The model under review builds one solid part; all positions refer to its coordinate system, in mm. A direction names the side the tool comes from. Round coordinates to 2 decimals unless told otherwise and drop trailing zeros. Write each loop counter-clockwise with the first axis right and the second up, starting at its lowest first coordinate (ties: lowest second). Pieces come first, ordered by that corner, then holes. Notation, with made-up numbers: (16, -31.5) - (75, -31.5) arc R27 ccw to (75, -7.5) - close; hole circle Ø2 at (-20, 51.25). An arc over 180 degrees is marked (long way). Use one line per item in the form item = value.
from build123d import *

# Parameters (mm, degrees)
BOSS_EXTRUDE1_DEPTH      = 2.54
SKETCH2_W                = 9.525
SKETCH2_H                = 38.1
BOSS_EXTRUDE2_DEPTH      = 15.875
BOSS_EXTRUDE3_DEPTH      = 5.08
M3_CLEARANCE_HOLE1_D     = 3.3
M3_CLEARANCE_HOLE1_DEPTH = 12.7
M3_CLEARANCE_HOLE1_TIP   = 0.991420021
SKETCH7_W                = 35.71875
SKETCH7_H                = 2.38125
CUT_EXTRUDE1_DEPTH       = 2.54
FILLET1_R                = 1.27
SKETCH8_R                = 3.4925
CUT_EXTRUDE2_DEPTH       = 10.16
CUT_EXTRUDE3_DEPTH       = 57.171484091
CUT_EXTRUDE3_DEPTH_BACK  = 57.171484091
SKETCH9_W                = 10.431111816
SKETCH9_H                = 47.706198334
FILLET3_R                = 1.27


with BuildPart() as part:
    # Sketch1 → Boss-Extrude1 (new body)
    with BuildSketch(Plane(origin=(0, 0, 0), x_dir=(1, 0, 0), z_dir=(0, 1, 0))):
        Polygon((0, 0), (38.1, 0), (38.1, 2.38125), (2.38125, 2.38125), (2.38125, 38.1), (0, 38.1), align=None)
    extrude(amount=BOSS_EXTRUDE1_DEPTH)

    # Sketch2 → Boss-Extrude2 (add)
    with BuildSketch(Plane(origin=(0, 2.54, 0), x_dir=(1, 0, 0), z_dir=(0, 1, 0))):
        with Locations((-4.7625, 19.05)):
            Rectangle(SKETCH2_W, SKETCH2_H)
        Polygon((0, 0), (-9.525, 0), (-9.525, -9.525), (38.1, -9.525), (38.1, 0), align=None)
    extrude(amount=-BOSS_EXTRUDE2_DEPTH)

    # Sketch3 → Boss-Extrude3 (add)
    with BuildSketch(Plane(origin=(0, -13.335, 0), x_dir=(-1, 0, 0), z_dir=(0, -1, 0))):
        Polygon((9.525, -9.525), (-38.1, -9.525), (-38.1, 18.373079092), (-18.373079092, 38.1), (9.525, 38.1), align=None)
    extrude(amount=BOSS_EXTRUDE3_DEPTH)

    # M3 Clearance Hole1
    with Locations(Plane(origin=(0, -18.415, 0), x_dir=(-1, 0, 0), z_dir=(0, -1, 0))):
        with Locations((-10, 32.5), (-32.5, 10)):
            Hole(M3_CLEARANCE_HOLE1_D / 2, depth=M3_CLEARANCE_HOLE1_DEPTH)
            with Locations((0, 0, -(M3_CLEARANCE_HOLE1_DEPTH + M3_CLEARANCE_HOLE1_TIP / 2))):  # 118° drill point
                Cone(0, M3_CLEARANCE_HOLE1_D / 2, M3_CLEARANCE_HOLE1_TIP, mode=Mode.SUBTRACT)

    # Sketch7 → Cut-Extrude1 (cut)
    with BuildSketch(Plane(origin=(0, 2.54, 0), x_dir=(1, 0, 0), z_dir=(0, 1, 0))):
        with Locations((20.240625, 1.190625)):
            Rectangle(SKETCH7_W, SKETCH7_H)
        Polygon((0, 0), (2.38125, 0), (2.38125, 2.38125), (2.38125, 38.1), (0, 38.1), align=None)
    extrude(amount=-CUT_EXTRUDE1_DEPTH, mode=Mode.SUBTRACT)

    # Fillet1
    fillet1_edges = [part.edges().sort_by_distance(p)[0] for p in [
        (38.1, 2.54, 4.7625),
        (0, -5.3975, -38.1),
        (-9.525, -7.9375, -38.1),
        (38.1, -5.3975, 0),
        (14.2875, 2.54, 9.525),
        (38.1, -7.9375, 9.525),
        (-9.525, -7.9375, 9.525),
        (-9.525, 2.54, -14.2875),
        (-9.525, -18.415, -14.2875),
        (14.2875, -18.415, 9.525),
        (-4.7625, 2.54, -38.1),
        (0, 2.54, -19.05),
        (19.05, 2.54, 0),
    ]]
    fillet(fillet1_edges, radius=FILLET1_R)

    # Sketch8 → Cut-Extrude2 (cut)
    with BuildSketch(Plane(origin=(0, -13.335, 0), x_dir=(1, 0, 0), z_dir=(0, 1, 0))):
        with Locations(Location((10, 32.5, 0), (0, 0, 270))):
            Circle(SKETCH8_R)
    extrude(amount=-CUT_EXTRUDE2_DEPTH, mode=Mode.SUBTRACT)

    # Sketch9 → Cut-Extrude3 (cut, two sides: drawn at the far end of the back side and taken through both)
    with BuildSketch(Plane(origin=(0, -13.335, 0), x_dir=(1, 0, 0), z_dir=(0, 1, 0)).offset(-CUT_EXTRUDE3_DEPTH_BACK)):
        with Locations((-9.978055908, 11.071900833)):
            Rectangle(SKETCH9_W, SKETCH9_H)
        Polygon((25.888370715, 34.925), (25.888370715, 38.1), (18.373079092, 38.1), (21.548079092, 34.925), align=None)
        with BuildLine():
            Line((21.548079092, 34.925), (18.373079092, 38.1))
            Line((18.373079092, 38.1), (-1.27, 38.1))
            ThreePointArc((-1.27, 38.1), (-0.371974388, 37.728025612), (0, 36.83))
            Line((0, 36.83), (0, 34.925))
            Line((0, 34.925), (7.486649398, 34.925))
            ThreePointArc((7.486649398, 34.925), (10, 35.9925), (12.513350602, 34.925))
            Line((12.513350602, 34.925), (21.548079092, 34.925))
        make_face()
        with BuildLine():
            ThreePointArc((0, 36.83), (-0.371974388, 37.728025612), (-1.27, 38.1))
            Line((-1.27, 38.1), (-15.193611816, 38.1))
            Line((-15.193611816, 38.1), (-15.193611816, 34.925))
            Line((-15.193611816, 34.925), (-4.7625, 34.925))
            Line((-4.7625, 34.925), (0, 34.925))
            Line((0, 34.925), (0, 36.83))
        make_face()
    extrude(amount=CUT_EXTRUDE3_DEPTH + CUT_EXTRUDE3_DEPTH_BACK, mode=Mode.SUBTRACT)

    # Fillet3
    fillet3_edges = [part.edges().sort_by_distance(p)[0] for p in [
        (-4.7625, 2.168025612, 9.153025612),
        (-4.7625, -7.9375, 9.525),
        (-0.371974388, 2.168025612, -34.925),
        (-3.01625, 2.54, -34.925),
        (-4.7625, -18.415, -13.335),
        (0, -6.0325, -34.925),
        (-4.7625, -18.043025612, 9.153025612),
        (-4.7625, -7.9375, -34.925),
        (-4.7625, 2.54, -13.335),
    ]]
    fillet(fillet3_edges, radius=FILLET3_R)


solid = part.part
(1) Insertion check: P1, Ø4.5, axis at x = 32.5, z = -10, coming from the +Y side (3 decimals); P2, Ø10, axis at y = -9.5, z = -28, coming from the +X side; P3, Ø2, axis at y = -13, z = -6.5, coming from the +X side; P4, Ø6.5, axis at x = 10, z = -32.5, coming from the -Y side. Each pin has a flat end and moves straight along its axis. Give the tip position at first contact, or say it passes through.
Geometry results:
P1 = -13.335
P2 = 31.68
P3 = 38.1
P4 = through
(2) Add section D-D on y = -4.5. Write out the cut boundary in (x, z) (1 decimal), then the cut area to 3 significant figures.
Geometry results:
outline = (-4.8, -33.7) arc R1.3 ccw to (-3.5, -34.9) - (-1.3, -34.9) arc R1.3 ccw to (0, -33.7) - (0, 0) - (36.8, 0) arc R1.3 ccw to (38.1, 1.3) - (38.1, 8.3) arc R1.3 ccw to (36.8, 9.5) - (-3.5, 9.5) arc R1.3 ccw to (-4.8, 8.3) - close
area = 573 mm2
(3) The part is to be moulded in two halves that separate along X. For faces 1 (the flat face through (18, -13.335, -17)), 2 (the cylindrical face through (9.89, -15.84, -29.01)), 3 (the cylindrical face through (-4.4, -18.033, -13.637)), 4 (the cylindrical face through (31.19, -15.84, -9)), say which applies: +X half, -X half, draft (parallel to the pull), parting line (faces both ways), or undercut.
Geometry results:
face_1 = draft
face_2 = undercut
face_3 = -X half
face_4 = undercut
(4) Add section C-C on x = 10. Write out the cut boundary in (y, z) (1 decimal).
Geometry results:
outline = (-18.4, -29) - (-13.3, -29) - (-13.3, 0) - (1.3, 0) arc R1.3 ccw to (2.5, 1.3) - (2.5, 8.3) arc R1.3 ccw to (1.3, 9.5) - (-17.1, 9.5) arc R1.3 ccw to (-18.4, 8.3) - close
(5) To check wall thickness, follow L1, parallel to X at y = -14.4, z = -10; L2, parallel to X at y = -4.5, z = -1.5; L3, parallel to Y at x = 13, z = -8 (3 decimals). State the ranges of each line that lie inside material, in increasing order.
Geometry results:
L1 = -4.76 to 30.85, 34.15 to 38.1
L2 = -4.76 to 0
L3 = -18.415 to -13.335
(6) Machinability: for faces 5 (the flat face through (16, -8, 9.525)), 6 (the flat face through (0, -6, -17)), which of the approach directions +Z, -Z, +X, -X, +Y, -Y give a long, thin tool a straight path to every point of the face, cutting with its end or side? Answer none if there is none.
Geometry results:
face_5 = +Z, +X, -X, +Y, -Y
face_6 = -Z, +X, +Y
